from build123d import *

# Parameters (mm, degrees)
F0_W     = 20
F0_H     = 20
F1_DEPTH = 20
F2_R     = 1
F3_R     = 5.1
F4_DEPTH = 20
F5_R     = 5.1
F6_DEPTH = 20


with BuildPart() as f1:
    # F0 (on Front) → F1 (new body)
    with BuildSketch(Plane.XZ):
        with Locations((-10, 30)):
            Rectangle(F0_W, F0_H)
        with Locations((10, 10)):
            Rectangle(F0_W, F0_H)
        Polygon((-20, 20), (0, 0), (0, 20), align=None)
        with BuildLine():
            ThreePointArc((-20, 20), (-14.1421356237, 5.8578643763), (0, 0))
            Line((0, 0), (-20, 20))
        make_face()
    extrude(amount=F1_DEPTH)

    # F2
    f2_edges = [f1.edges().sort_by_distance(p)[0] for p in [
        (0, -20, 30),
        (0, -10, 40),
        (-10, -20, 40),
        (-20, -10, 40),
        (10, -20, 20),
        (10, 0, 20),
        (20, -10, 20),
        (20, -20, 10),
        (20, 0, 10),
        (20, -10, 0),
        (10, -20, 0),
        (-20, -20, 30),
        (0, 0, 30),
        (-10, 0, 40),
        (-20, 0, 30),
        (10, 0, 0),
        (-14.142136, -20, 5.857864),
        (0, -10, 20),
    ]]
    fillet(f2_edges, radius=F2_R)

    # F3 (on face) → F4 (cut)
    with BuildSketch(Plane.XY.offset(40)):
        with Locations((-10, -10)):
            Circle(F3_R)
    extrude(amount=-F4_DEPTH, mode=Mode.SUBTRACT)

    # F5 (on face) → F6 (cut)
    with BuildSketch(Plane.YZ.offset(20)):
        with Locations((-10, 10)):
            Circle(F5_R)
    extrude(amount=-F6_DEPTH, mode=Mode.SUBTRACT)


solid = f1.part
CAD build for the part. Positions are in the model's coordinates, mm. A direction names the side the tool comes from. Round coordinates to 2 decimals unless told otherwise and drop trailing zeros. Write each loop counter-clockwise with the first axis right and the second up, starting at its lowest first coordinate (ties: lowest second). Pieces come first, ordered by that corner, then holes. Notation, with made-up numbers: (-34, 55) -> (-15, 55) arc R30 ccw to (-15, 89) -> close; hole circle Ø11 at (16.25, 20). An arc over 180 degrees is marked (long way). Answer as a JSON object with one key per item and string values.
(1) Band-saw the part on B-B, the plane z = 34. List the corners of the cut face in (x, y).
Reported:
{"outline": "(-20, -19) arc R1 ccw to (-19, -20) -> (-1, -20) arc R1 ccw to (0, -19) -> (0, -1) arc R1 ccw to (-1, 0) -> (-19, 0) arc R1 ccw to (-20, -1) -> close; hole circle Ø10.2 at (-10, -10)"}
(2) Probe probe 1 along Y at (x, z) = (-10, 26.25); probe 2 along Z at (x, y) = (7.5, -10); probe 3 along Y at (x, z) = (-6, 25). List the from-to ranges inside material, lowest first. Write a range as [from, to].
Reported:
{"probe 1": "y = [-20, -15.1], [-4.9, 0]", "probe 2": "z = [0, 4.9], [15.1, 20]", "probe 3": "y = [-20, -13.16], [-6.84, 0]"}
(3) Band-saw the part on C-C, the plane y = -1.5. List the corners of the cut face in (x, z), then the cut area to 3 significant figures.
Reported:
{"outline": "(-20, 20) arc R20 ccw to (0, 0) -> (19, 0) arc R1 ccw to (20, 1) -> (20, 19) arc R1 ccw to (19, 20) -> (1, 20) arc R1 cw to (0, 21) -> (0, 39) arc R1 ccw to (-1, 40) -> (-19, 40) arc R1 ccw to (-20, 39) -> close", "area": "1,110 mm^2"}
(4) Two-plate mould, pull along Y, no slides. Class faces 1 (the face through (0, -10, 10)), 2 (the face through (19.715, -0.301, 10.126)), 3 (the face through (10, -10, 20)): +Y half, -Y half, draft (parallel to the pull), parting line (faces both ways), or undercut.
Reported:
{"face 1": "undercut", "face 2": "+Y half", "face 3": "draft"}
(5) Pin check, flat tips, straight feed: P1, Ø4, axis at x = 4, y = -16, coming from the +Z side; P2, Ø1, axis at y = -15.5, z = 18, coming from the -X side; P3, Ø4, axis at y = -10.5, z = 7.5, coming from the +X side. Stop position of each tip, or through.
Reported:
{"P1": "stops at z = 20", "P2": "stops at x = -19.94", "P3": "stops at x = 0"}
(6) Which spindle directions (+Z, -Z, +X, -X, +Y, -Y) get a long thin tool onto all of the face, cutting with end or side? Do faces 4 (the face through (10.126, -0.301, 19.715)), 5 (the face through (-5.136, -8.468, 30.14)), 6 (the face through (10.126, -19.699, 19.715)). Say none if no direction does.
Reported:
{"face 4": "+Z, +X, +Y", "face 5": "+Z", "face 6": "+Z, +X, -Y"}
(7) Band-saw the part on A-A, the plane x = 17. List the corners of the cut face in (y, z), then the cut area to 3 significant figures.
Reported:
{"outline": "(-20, 1) arc R1 ccw to (-19, 0) -> (-1, 0) arc R1 ccw to (0, 1) -> (0, 19) arc R1 ccw to (-1, 20) -> (-19, 20) arc R1 ccw to (-20, 19) -> close; hole circle Ø10.2 at (-10, 10)", "area": "317 mm^2"}
(8) Band-saw the part on D-D, the plane y = -10. List the corners of the cut face in (x, z).
Reported:
{"outline": "(-20, 20) arc R20 ccw to (0, 0) -> (19, 0) arc R1 ccw to (20, 1) -> (20, 4.9) -> (0, 4.9) -> (0, 15.1) -> (20, 15.1) -> (20, 19) arc R1 ccw to (19, 20) -> (1, 20) arc R1 cw to (0, 21) -> (0, 39) arc R1 ccw to (-1, 40) -> (-4.9, 40) -> (-4.9, 20) -> (-15.1, 20) -> (-15.1, 40) -> (-19, 40) arc R1 ccw to (-20, 39) -> close"}
